The model under review builds one solid part; all positions refer to its coordinate system, in mm. A direction names the side the tool comes from. Round coordinates to 2 decimals unless told otherwise and drop trailing zeros. Write each loop counter-clockwise with the first axis right and the second up, starting at its lowest first coordinate (ties: lowest second). Pieces come first, ordered by that corner, then holes. Notation, with made-up numbers: (-23.5, -26.75) - (15.5, -26.75) arc R16 cw to (15.5, 4.25) - close; hole circle Ø4 at (63, 49.25). An arc over 180 degrees is marked (long way). Return JSON: item names as keys, results as strings.
from build123d import *

# Parameters (mm, degrees)
SKETCH1_W               = 169
SKETCH1_H               = 89
SKETCH1_W_2             = 161
SKETCH1_H_2             = 81
BOSS_EXTRUDE1_DEPTH     = 15
SKETCH2_W               = 169
SKETCH2_H               = 89
SKETCH2_W_2             = 43
SKETCH2_H_2             = 57
SKETCH2_W_3             = 41
SKETCH2_W_4             = 35
BOSS_EXTRUDE2_DEPTH     = 3
SKETCH4_R               = 1.5
CUT_EXTRUDE1_DEPTH      = 13
SKETCH5_R               = 2.5
CUT_EXTRUDE2_DEPTH      = 2
SKETCH6_R               = 1.5
CUT_EXTRUDE3_DEPTH      = 10
SKETCH8_R               = 1.5
CUT_EXTRUDE4_DEPTH      = 4
MIRROR2_COPY_1_SKETCH_R = 1.5
MIRROR2_COPY_1_DEPTH    = 4
SKETCH10_R              = 1.35
CUT_EXTRUDE5_DEPTH      = 4
SKETCH11_W              = 25
SKETCH11_H              = 10
BOSS_EXTRUDE3_DEPTH     = 10
SKETCH12_R              = 1.5
CUT_EXTRUDE6_DEPTH      = 10


with BuildPart() as part:
    # Sketch1 → Boss-Extrude1 (new body)
    with BuildSketch(Plane(origin=(0, 0, 0), x_dir=(1, 0, 0), z_dir=(0, 1, 0))):
        Rectangle(SKETCH1_W, SKETCH1_H)
        Rectangle(SKETCH1_W_2, SKETCH1_H_2, mode=Mode.SUBTRACT)
    extrude(amount=BOSS_EXTRUDE1_DEPTH)

    # Sketch2 → Boss-Extrude2 (add)
    with BuildSketch(Plane(origin=(0, 0, 0), x_dir=(-1, 0, 0), z_dir=(0, -1, 0))):
        Rectangle(SKETCH2_W, SKETCH2_H)
        with Locations((45, 0)):
            Rectangle(SKETCH2_W_2, SKETCH2_H_2, mode=Mode.SUBTRACT)
        with Locations((-46, 0)):
            Rectangle(SKETCH2_W_3, SKETCH2_H_2, mode=Mode.SUBTRACT)
        with Locations((-1, 0)):
            Rectangle(SKETCH2_W_4, SKETCH2_H_2, mode=Mode.SUBTRACT)
    extrude(amount=BOSS_EXTRUDE2_DEPTH)

    # Sketch4 → Cut-Extrude1 (cut)
    with BuildSketch(Plane(origin=(-80.5, 0, 0), x_dir=(0, 0, -1), z_dir=(1, 0, 0))):
        with Locations((-25, 6.604468408)):
            Circle(SKETCH4_R)
        with Locations((25, 6.604468408)):
            Circle(SKETCH4_R)
    extrude(amount=-CUT_EXTRUDE1_DEPTH, mode=Mode.SUBTRACT)

    # Sketch5 → Cut-Extrude2 (cut)
    with BuildSketch(Plane(origin=(-80.5, 0, 0), x_dir=(0, 0, -1), z_dir=(1, 0, 0))):
        with Locations((-25, 6.604468408)):
            Circle(SKETCH5_R)
        with Locations((25, 6.604468408)):
            Circle(SKETCH5_R)
    extrude(amount=-CUT_EXTRUDE2_DEPTH, mode=Mode.SUBTRACT)

    # Sketch6 → Cut-Extrude3 (cut)
    with BuildSketch(Plane(origin=(0, -3, 0), x_dir=(-1, 0, 0), z_dir=(0, -1, 0))):
        with Locations(Location((-9.5, 37.5, 0), (0, 0, 90))):
            Circle(SKETCH6_R)
        with Locations(Location((-64.5, 37.5, 0), (0, 0, 90))):
            Circle(SKETCH6_R)
    extrude(amount=-CUT_EXTRUDE3_DEPTH, mode=Mode.SUBTRACT)

    # Sketch8 → Cut-Extrude4 (cut)
    with BuildSketch(Plane(origin=(0, 0, 0), x_dir=(1, 0, 0), z_dir=(0, 1, 0))):
        with Locations(Location((-62.5, 32.5, 0), (0, 0, 270))):
            Circle(SKETCH8_R)
    cut_extrude4 = extrude(amount=-CUT_EXTRUDE4_DEPTH, mode=Mode.SUBTRACT)

    # Mirror1: Cut-Extrude4 across plane
    add(cut_extrude4.mirror(Plane(origin=(0, 0, 0), x_dir=(0, 0, 1), z_dir=(1, 0, 0))), mode=Mode.SUBTRACT)

    # Mirror2: Cut-Extrude4 across plane
    add(cut_extrude4.mirror(Plane.XY), mode=Mode.SUBTRACT)

    # Mirror2 copy 1 sketch → Mirror2 copy 1 (cut)
    with BuildSketch(Plane(origin=(0, 0, 0), x_dir=(-1, 0, 0), z_dir=(0, 1, 0))):
        with Locations(Location((-62.5, 32.5, 0), (0, 0, 270))):
            Circle(MIRROR2_COPY_1_SKETCH_R)
    extrude(amount=-MIRROR2_COPY_1_DEPTH, mode=Mode.SUBTRACT)

    # Sketch10 → Cut-Extrude5 (cut)
    with BuildSketch(Plane.XZ.offset(3)):
        with Locations(Location((72.5, 15.5, 0), (0, 0, 270))):
            Circle(SKETCH10_R)
        with Locations(Location((-72.5, -15.5, 0), (0, 0, 270))):
            Circle(SKETCH10_R)
    extrude(amount=-CUT_EXTRUDE5_DEPTH, mode=Mode.SUBTRACT)

    # Sketch11 → Boss-Extrude3 (add)
    with BuildSketch(Plane.XZ.offset(3)):
        with Locations((72, 49.5)):
            Rectangle(SKETCH11_W, SKETCH11_H)
    boss_extrude3 = extrude(amount=-BOSS_EXTRUDE3_DEPTH)

    # Sketch12 → Cut-Extrude6 (cut)
    with BuildSketch(Plane.XZ.offset(3)):
        with Locations(Location((64.5, 49.5, 0), (0, 0, 270))):
            Circle(SKETCH12_R)
        with Locations(Location((79.5, 49.5, 0), (0, 0, 270))):
            Circle(SKETCH12_R)
    cut_extrude6 = extrude(amount=-CUT_EXTRUDE6_DEPTH, mode=Mode.SUBTRACT)

    # Mirror3: Boss-Extrude3, Cut-Extrude6 across plane
    add(boss_extrude3.mirror(Plane.XY))
    add(cut_extrude6.mirror(Plane.XY), mode=Mode.SUBTRACT)


solid = part.part
(1) Mouldability with a two-part tool opening along Y and no side actions: class faces 1 (the flat face through (59.5, 2, -49)), 2 (the flat face through (-17, 0, -1)), 3 (the cylindrical face through (-81.5, 6.7, -22.5)) as released by +Y, released by -Y, zero draft, split by the parting line, or undercut.
Filled in:
{"face 1": "zero draft", "face 2": "released by +Y", "face 3": "undercut"}
(2) Wall thickness on line 1 (X direction, y = -0.8, z = -37.5); line 2 (X direction, y = -1.6, z = 32.5); line 3 (X direction, y = 8.5, z = 11): over which ranges is each line inside the solid? List them lowest first.
Filled in:
{"line 1": "x = -84.5 to 8, 11 to 63, 66 to 84.5", "line 2": "x = -84.5 to -64, -61 to 61, 64 to 84.5", "line 3": "x = -84.5 to -80.5, 80.5 to 84.5"}
(3) Add section B-B (y = 12). Write out the cut boundary in (x, z), plus the area to 3 significant figures.
Filled in:
{"outline": "(-84.5, -44.5) - (84.5, -44.5) - (84.5, 44.5) - (-84.5, 44.5) - close; hole (-80.5, -40.5) - (80.5, -40.5) - (80.5, 40.5) - (-80.5, 40.5) - close", "area": "2,000 mm2"}
(4) Clearance check with flat-ended pins moving along their axes: pin 1 Ø0.9 at (x, y) = (-43, -2) entering from -Z; pin 2 Ø4.5 at (x, y) = (-26.5, 10) entering from +Z; pin 3 Ø3 at (x, z) = (-72.5, -15.5) entering from +Y; pin 4 Ø2.5 at (x, z) = (64.5, 49.5) entering from -Y. State where each tip first meets the part, or that it passes through.
Filled in:
{"pin 1": "stops at z = -44.5", "pin 2": "stops at z = 44.5", "pin 3": "stops at y = 0", "pin 4": "passes through"}
(5) Add section A-A (x = -44.5). Write out the cut boundary in (y, z).
Filled in:
{"outline": "(-3, -44.5) - (15, -44.5) - (15, -40.5) - (0, -40.5) - (0, -28.5) - (-3, -28.5) - close; (-3, 28.5) - (0, 28.5) - (0, 40.5) - (15, 40.5) - (15, 44.5) - (-3, 44.5) - close"}
(6) For faces 4 (the flat face through (59.5, 2, 49)), 5 (the flat face through (-82.5, 7, -27)), 6 (the flat face through (-80.5, 7, 1)), list the 3-axis set-ups (+Z, -Z, +X, -X, +Y, -Y) from which the entire face can be reached by the end or side of a thin tool; tool diameter is ignored.
Filled in:
{"face 4": "+Z, -X, +Y, -Y", "face 5": "none", "face 6": "+Y"}
